```python
from build123d import *

# Parameters (mm, degrees)
SKETCH_1_W                   = 25
SKETCH_1_H                   = 4.7
SKETCH_1_R                   = 1.1
EXTRUDE_1_DEPTH              = 2.5
HOLE_WIZARD_M2_1_D           = 2
HOLE_WIZARD_M2_1_CSINK_D     = 4.1
HOLE_WIZARD_M2_1_CSINK_ANGLE = 90
EXTRUDE_2_DEPTH              = 2.5
SKETCH1_R                    = 0.85
EXTRUDE1_DEPTH               = 10
SKETCH3_R                    = 2.05
EXTRUDE2_DEPTH               = 10
EXTRUDE4_DEPTH               = 2.5
EXTRUDE5_DEPTH               = 10
FILLET1_R                    = 2
FILLET2_R                    = 1
FILLET3_R                    = 2


with BuildPart() as part:
    # 草图1 → 凸台-拉伸1 (new body)
    with BuildSketch(Plane(origin=(0, 0, 0), x_dir=(0, 0, -1), z_dir=(1, 0, 0))):
        Rectangle(SKETCH_1_W, SKETCH_1_H)
        with Locations((9.5, 0)):
            Circle(SKETCH_1_R, mode=Mode.SUBTRACT)
        with Locations((-9.5, 0)):
            Circle(SKETCH_1_R, mode=Mode.SUBTRACT)
    extrude(amount=EXTRUDE_1_DEPTH)

    # M2 平头机械螺钉的锥形沉头孔1 (through all)
    with Locations(Plane(origin=(2.5, 0, 9.5), x_dir=(0, 0, 1), z_dir=(1, 0, 0))):
        with Locations((0, 0), (-19, 0)):
            CounterSinkHole(HOLE_WIZARD_M2_1_D / 2, HOLE_WIZARD_M2_1_CSINK_D / 2, counter_sink_angle=HOLE_WIZARD_M2_1_CSINK_ANGLE)

    # 草图3 → 凸台-拉伸2 (add, symmetric)
    with BuildSketch(Plane.XY):
        Polygon((0, -2.35), (2.5, -2.35), (2.5, -22.35), (-5.5, -22.35), (-5.5, -18.35), (-2, -18.35), (0, -16.35), align=None)
    extrude(amount=EXTRUDE_2_DEPTH, both=True)

    # Sketch1 → Extrude1 (cut)
    with BuildSketch(Plane(origin=(0, -18.35, 0), x_dir=(1, 0, 0), z_dir=(0, 1, 0))):
        with Locations(Location((-3, 0, 0), (0, 0, 270))):  # turned: the seam where the file's is
            Circle(SKETCH1_R)
    extrude(amount=-EXTRUDE1_DEPTH, mode=Mode.SUBTRACT)

    # Sketch2 → CSK for M2 Flat Head Machine Screw1 (revolve, cut)
    with BuildSketch(Plane(origin=(-3, -18.35, 0), x_dir=(0, 0, 1), z_dir=(1, 0, 0))):
        Polygon((0, 0), (0, 4.000025), (1, 4.000025), (1, 1.05), (2.05, 0), align=None)
    revolve(axis=Axis((-3, -12, 0), (0, -1, 0)), mode=Mode.SUBTRACT)

    # Sketch3 → Extrude2 (cut)
    with BuildSketch(Plane(origin=(0, -18.35, 0), x_dir=(1, 0, 0), z_dir=(0, 1, 0))):
        with Locations((-3, 0)):
            Circle(SKETCH3_R)
    extrude(amount=EXTRUDE2_DEPTH, mode=Mode.SUBTRACT)

    # Sketch6 → Extrude4 (add)
    with BuildSketch(Plane(origin=(2.5, 0, 0), x_dir=(0, 0, -1), z_dir=(1, 0, 0))):
        Polygon((-12.5, -2.35), (-2.5, -2.35), (-2.5, -14.35), (-12.5, -4.35), align=None)
        Polygon((12.5, -4.35), (12.5, -2.35), (2.5, -2.35), (2.5, -14.35), align=None)
    extrude(amount=-EXTRUDE4_DEPTH)

    # Sketch7 → Extrude5 (cut)
    with BuildSketch(Plane(origin=(2.5, 0, 0), x_dir=(0, 0, -1), z_dir=(1, 0, 0))):
        with BuildLine():
            Line((-4, -4.5), (4, -4.5))
            ThreePointArc((4, -4.5), (5, -5.5), (4, -6.5))
            Line((4, -6.5), (-4, -6.5))
            ThreePointArc((-4, -6.5), (-5, -5.5), (-4, -4.5))
        make_face()
    extrude(amount=-EXTRUDE5_DEPTH, mode=Mode.SUBTRACT)

    # Fillet1
    fillet1_edges = [part.edges().sort_by_distance(p)[0] for p in [
        (1.25, -4.35, -12.5),
        (1.25, -14.35, -2.5),
        (1.25, -14.35, 2.5),
        (1.25, -4.35, 12.5),
        (1.25, 2.35, -12.5),
        (1.25, 2.35, 12.5),
    ]]
    fillet(fillet1_edges, radius=FILLET1_R)

    # Fillet2
    fillet2_edges = [part.edges().sort_by_distance(p)[0] for p in [
        (-5.5, -20.35, -2.5),
        (-5.5, -20.35, 2.5),
    ]]
    fillet(fillet2_edges, radius=FILLET2_R)

    # Fillet3
    fillet3_edges = [part.edges().sort_by_distance(p)[0] for p in [
        (2.5, -22.35, 0),
    ]]
    fillet(fillet3_edges, radius=FILLET3_R)


solid = part.part
```
The listing builds one solid part. Answer for the finished solid, in the listing's coordinates (mm). A direction names the side the tool comes from. Give positions to 0.01 mm unless a question says otherwise; leave off trailing zeros. Order: outer loops, then holes, each group sorted by start corner. A loop starts at its lowest first (then second) coordinate and runs counter-clockwise, first axis right, second up. Notation, with made-up numbers: (-33.75, -15) -> (-10.75, -15) arc R22 cw to (-10.75, 11) -> close; hole circle Ø11 at (-3, 29.25). An arc over 180 degrees is marked (long way). One line per item, written item: value.
1) Flat-ended cylindrical pins translate along their axes: P1, Ø4, axis at x = -3.5, z = -3.5, coming from the +Y side; P2, Ø2, axis at y = 0, z = 9.5, coming from the +X side; P3, Ø9.5, axis at y = -6.5, z = -4.5, coming from the -X side; P4, Ø3, axis at x = -4.5, z = 1, coming from the +Y side. Find the tip coordinate at first contact, or state that the pin passes through.
Reported:
P1: stops at y = -18.12
P2: passes through
P3: stops at x = 0
P4: stops at y = -18.35
2) Determine the mould class of faces 1 (the flat face through (-1.8, -22.35, 0)), 2 (the cylindrical face through (1.27, 1.75, 11.93)), 3 (the cylindrical face through (0.764, -0.421, -10.516)), 4 (the flat face through (0, -20, -2.5)) for opening direction Y: pulls with the +Y half, pulls with the -Y half, needs draft (parallel to the pull), parting line crosses it, or undercut.
Reported:
face 1: pulls with the -Y half
face 2: pulls with the +Y half
face 3: undercut
face 4: needs draft
3) Find section B-B, the plane z = 3.5. Determine the outline of the cut face in (x, y), plus the area to 4 significant figures.
Reported:
outline: (0, -13.35) -> (2.5, -13.35) -> (2.5, -6.5) -> (0, -6.5) -> close; (0, -4.5) -> (2.5, -4.5) -> (2.5, 2.35) -> (0, 2.35) -> close
area: 34.25 mm^2
4) Find the intervals of material crossed by line 1 (X direction, y = -20.2, z = 0); line 2 (Z direction, x = -3, y = -21); line 3 (Y direction, x = 0.25, z = -1), in increasing order.
Reported:
line 1: x = -5.5 to -4, -2 to 2.5
line 2: z = -2.5 to -1, 1 to 2.5
line 3: y = -22.35 to -6.5, -4.5 to 2.35
5) Find section C-C, the plane y = 0. Determine the outline of the cut face in (x, z), plus the area to 3 significant figures.
Reported:
outline: (0, -12.5) -> (2.5, -12.5) -> (2.5, -11.55) -> (1.55, -10.6) -> (0, -10.6) -> close; (0, -8.4) -> (1.55, -8.4) -> (2.5, -7.45) -> (2.5, 7.45) -> (1.55, 8.4) -> (0, 8.4) -> close; (0, 10.6) -> (1.55, 10.6) -> (2.5, 11.55) -> (2.5, 12.5) -> (0, 12.5) -> close
area: 49.7 mm^2
6) A tool of negligible diameter and unlimited length cuts with its end or side. For faces 5 (the flat face through (1, -2, -12.5)), 6 (the flat face through (1, -6.5, 0)), 7 (the flat face through (0, -20, 2.5)), from which of +Z, -Z, +X, -X, +Y, -Y can it reach the whole face along a straight path? Write none if from no direction.
Reported:
face 5: -Z, +X, -X, +Y, -Y
face 6: +X, -X
face 7: +Z, +X, -X, -Y
7) Find section D-D, the plane z = -9.5. Determine the outline of the cut face in (x, y), plus the area to 3 significant figures.
Reported:
outline: (0, -7.35) -> (2.5, -7.35) -> (2.5, -2.05) -> (1.55, -1.1) -> (0, -1.1) -> close; (0, 1.1) -> (1.55, 1.1) -> (2.5, 2.05) -> (2.5, 2.35) -> (0, 2.35) -> close
area: 17.8 mm^2
8) Find section A-A, the plane x = -3. Determine the outline of the cut face in (y, z).
Reported:
outline: (-22.35, -2.5) -> (-18.35, -2.5) -> (-18.35, -2.05) -> (-19.4, -1) -> (-22.35, -1) -> close; (-22.35, 1) -> (-19.4, 1) -> (-18.35, 2.05) -> (-18.35, 2.5) -> (-22.35, 2.5) -> close
